Verification items for the finished model (mm, model axes). Round coordinates to 2 decimals unless told otherwise and drop trailing zeros. Write each loop counter-clockwise with the first axis right and the second up, starting at its lowest first coordinate (ties: lowest second). Pieces come first, ordered by that corner, then holes. Notation, with made-up numbers: (62.5, 73.25) - (90.5, 73.25) arc R15 ccw to (90.5, 87.25) - close; hole circle Ø11 at (31.5, 8.5). An arc over 180 degrees is marked (long way). Answer as a JSON object with one key per item and string values.
```python
from build123d import *

# Parameters (mm, degrees)
EXTRUDE1_DEPTH     = 4.7625
FILLET3_R          = 0.127
CUT_EXTRUDE2_DEPTH = 4.7625


# Read off the part's stored shape, not the designer's step: Cut-Extrude2
with BuildPart() as part:
    # Sketch1 → Extrude1 (new body)
    with BuildSketch(Plane.XY):
        with BuildLine():
            Line((-12.598784067, -1.6002), (12.598784067, -1.6002))
            ThreePointArc((12.598784067, -1.6002), (0, -12.7), (-12.598784067, -1.6002))
        make_face()
    extrude(amount=EXTRUDE1_DEPTH)

    # Fillet3
    fillet3_edges = [part.edges().sort_by_distance(p)[0] for p in [
        (0, -1.6002, 0),
        (0, -12.7, 0),
        (0, -12.7, 4.7625),
        (-12.598784067, -1.6002, 2.38125),
        (12.598784067, -1.6002, 2.38125),
        (0, -1.6002, 4.7625),
    ]]
    fillet(fillet3_edges, radius=FILLET3_R)

    # Cut-Extrude2 outline → Cut-Extrude2 (cut)
    with BuildSketch(Plane.XY):
        with BuildLine():
            Line((3.087432428, -12.319), (-3.087432428, -12.319))
            ThreePointArc((-3.087432428, -12.319), (0, -12.7), (3.087432428, -12.319))
        make_face()
    extrude(amount=CUT_EXTRUDE2_DEPTH, mode=Mode.SUBTRACT)


solid = part.part
```
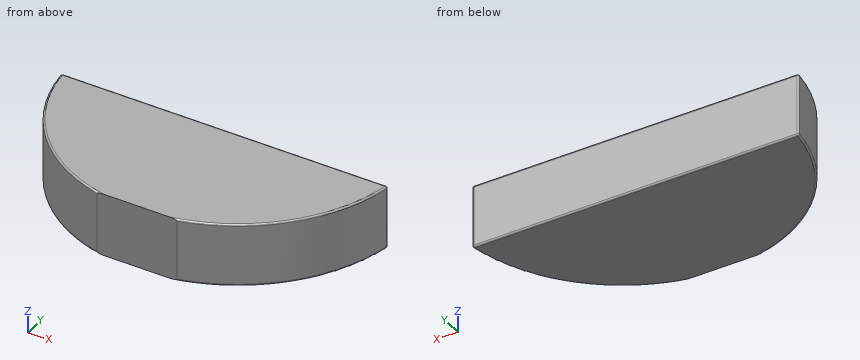
Q1. Section check A-A, the plane z = 2.15. Record the cut outline in (x, y), then the cut area to 3 significant figures.
Geometry check:
{"outline": "(-12.58, -1.74) arc R12.7 ccw to (-3.09, -12.32) - (3.09, -12.32) arc R12.7 ccw to (12.58, -1.74) arc R0.13 ccw to (12.45, -1.6) - (-12.45, -1.6) arc R0.13 ccw to start", "area": "211 mm2"}
Q2. Material ranges on line 1 along X through (y, z) = (-2.5, 2.15); line 2 along Y through (x, z) = (-4, 3.05); line 3 along X through (y, z) = (-9.25, 1.85), recorded low to high. Write a range as [from, to].
Geometry check:
{"line 1": "x = [-12.45, 12.45]", "line 2": "y = [-12.05, -1.6]", "line 3": "x = [-8.7, 8.7]"}
Q3. Gauge pin test, flat ends, axial feed: P1, Ø1.5, axis at y = -9.5, z = 2, coming from the +X side; P2, Ø1.5, axis at y = -9, z = 0.5, coming from the -X side; P3, Ø2, axis at y = -5, z = 3, coming from the -X side. Record the tip position at first contact, or that the pin passes through.
Geometry check:
{"P1": "stops at x = 9.2", "P2": "stops at x = -9.66", "P3": "stops at x = -12.05"}
